```python
from build123d import *

# Parameters (mm, degrees)
BOSS_EXTRUDE1_DEPTH = 1.5875
SKETCH3_R           = 2.032
CUT_EXTRUDE1_DEPTH  = 80.437624756


with BuildPart() as part:
    # Sketch2 → Boss-Extrude1 (new body)
    with BuildSketch(Plane(origin=(0, 0, 0), x_dir=(1, 0, 0), z_dir=(0, 1, 0))):
        with BuildLine():
            Line((44.536177097, 1.424957669), (-0.512568563, -7.225605856))
            ThreePointArc((-0.512568563, -7.225605856), (-3.031855718, -10.942384331), (0.684922757, -13.461671486))
            Line((0.684922757, -13.461671486), (45.733668417, -4.811107961))
            ThreePointArc((45.733668417, -4.811107961), (60.383311669, -6.347108045), (71.717083543, -15.755453212))
            ThreePointArc((71.717083543, -15.755453212), (76.116254433, -16.654644785), (77.015446005, -12.255473895))
            ThreePointArc((77.015446005, -12.255473895), (62.848231163, -0.495042436), (44.536177097, 1.424957669))
        make_face()
    extrude(amount=BOSS_EXTRUDE1_DEPTH)

    # Sketch3 → Cut-Extrude1 (cut, through all)
    with BuildSketch(Plane(origin=(0, 1.5875, 0), x_dir=(1, 0, 0), z_dir=(0, 1, 0))):
        with Locations(Location((51.871233594, -1.212563202, 0), (0, 0, 270))):
            Circle(SKETCH3_R)
    extrude(amount=-CUT_EXTRUDE1_DEPTH, mode=Mode.SUBTRACT)


solid = part.part
```
Verification items for the finished model (mm, model axes). A direction names the side the tool comes from. Give positions to 0.01 mm unless a question says otherwise; leave off trailing zeros. Loops run counter-clockwise (first coordinate to the right, second up) from the corner with the lowest first, then second, coordinate; pieces in that order, holes last.
1. Section check C-C, the plane x = 23. Enter the section's corners in (y, z), then the cut area to 3 significant figures.
2. Mould release check, pull along Z, two halves, no side actions. Record for faces 1 (the cylindrical face through (60.19, 0.783, 6.267)), 2 (the cylindrical face through (53.886, 0.805, 0.948)), 3 (the flat face through (22.33, 0.78, 2.84)): released by +Z, released by -Z, zero draft, split by the parting line, or undercut.
3. Section check B-B, the plane y = 1. Enter the section's corners in (x, z) (3 decimals), then the cut area to 3 significant figures.
4. Set-up check for faces 4 (the flat face through (22.894, 0.783, 9.197)), 5 (the flat face through (37, 1.588, 5)): record each of +Z, -Z, +X, -X, +Y, -Y from which the full face is reachable in a straight line by a thin tool's end or side.
5. Section check A-A, the plane z = 0. Enter the section's corners in (x, y), then the cut area to 3 significant figures.
6. Section check D-D, the plane x = 47.5. Enter the section's corners in (y, z), then the cut area to 3 significant figures.
7. Thickness scan on line 1 (X direction, y = 0.6, z = 13.75); line 2 (Z direction, x = 63, y = 1.5); line 3 (Z direction, x = 46.5, y = 1.15). Record the ranges inside material, lowest first.
Geometry says:
1. outline: (0, 2.71) - (1.59, 2.71) - (1.59, 9.18) - (0, 9.18) - close
1. area: 10.3 mm2
2. face 1: released by +Z
2. face 2: undercut
2. face 3: released by -Z
3. outline: (-0.513, 7.226) - (44.536, -1.425) arc R31.75 ccw to (77.015, 12.255) arc R3.175 ccw to (71.717, 15.755) arc R25.4 cw to (45.734, 4.811) - (0.685, 13.462) arc R3.175 ccw to start; hole circle Ø4.064 at (51.871, 1.213)
3. area: 524 mm2
4. face 4: +Z, +Y, -Y
4. face 5: +Z, -Z, +X, -X, +Y
5. outline: (37.12, 0) - (50.24, 0) - (50.24, 1.59) - (37.12, 1.59) - close; (53.5, 0) - (61.6, 0) - (61.6, 1.59) - (53.5, 1.59) - close
5. area: 33.7 mm2
6. outline: (0, -1.85) - (1.59, -1.85) - (1.59, 4.54) - (0, 4.54) - close
6. area: 10.1 mm2
7. line 1: x = 70.25 to 77.53
7. line 2: z = 0.56 to 7.63
7. line 3: z = -1.74 to 4.68
